The listing builds one solid part. Answer for the finished solid, in the listing's coordinates (mm). A direction names the side the tool comes from. Coordinates: 2 decimals unless noted, no trailing zeros.
from build123d import *

# Parameters (mm, degrees)
F0_W     = 76.2
F0_H     = 76.2
F1_DEPTH = 76.2
F2_W     = 76.2
F2_H     = 76.2
F3_DEPTH = 25.4
F4_W     = 101.6
F4_H     = 76.2
F5_DEPTH = 25.4
F6_W     = 101.6
F6_H     = 101.6
F7_DEPTH = 25.4


with BuildPart() as f1:
    # F0 (on Front) → F1 (new body)
    with BuildSketch(Plane.XZ):
        with Locations((-4.5091081411, 9.3812153666)):
            Rectangle(F0_W, F0_H)
    extrude(amount=F1_DEPTH)

    # F2 (on face) → F3 (join)
    with BuildSketch(Plane.YZ.offset(33.5908918589)):
        with Locations((-38.1, 9.3812153666)):
            Rectangle(F2_W, F2_H)
        with BuildLine():
            Line((-40.5894218998, 3.1841353355), (-54.3512732325, 3.1841353355))
            Line((-54.3512732325, 3.1841353355), (-54.3512732325, -24.2241639644))
            Line((-54.3512732325, -24.2241639644), (-62.0111716158, -24.2241639644))
            Line((-62.0111716158, -24.2241639644), (-62.0111716158, 41.6855831415))
            Line((-62.0111716158, 41.6855831415), (-43.9361194985, 41.6855831415))
            add(Edge.make_bspline(
                [(-43.9361194985, 41.6855831415), (-31.8043407032, 41.6855831415), (-26.0125342985, 37.0405976812)],
                knots=[0, 0, 0, 1, 1, 1], degree=2))
            add(Edge.make_bspline(
                [(-26.0125342985, 37.0405976812), (-20.2207278938, 32.3956122209), (-20.2207278938, 23.0623650382)],
                knots=[0, 0, 0, 1, 1, 1], degree=2))
            add(Edge.make_bspline(
                [(-20.2207278938, 23.0623650382), (-20.2207278938, 9.9929338984), (-33.4776895025, 5.3912247002)],
                knots=[0, 0, 0, 1, 1, 1], degree=2))
            Line((-33.4776895025, 5.3912247002), (-15.5757424335, -24.2241639644))
            Line((-15.5757424335, -24.2241639644), (-24.6349066232, -24.2241639644))
            Line((-24.6349066232, -24.2241639644), (-40.5894218998, 3.1841353355))
        make_face(mode=Mode.SUBTRACT)
    extrude(amount=F3_DEPTH)

    # F4 (on face) → F5 (join)
    with BuildSketch(Plane.XZ.offset(76.2)):
        with Locations((8.1908918589, 9.3812153666)):
            Rectangle(F4_W, F4_H)
        Polygon((19.8698597014, -23.9472966641), (12.0777951104, -23.9472966641), (4.0165501062, -3.3620787536), (-21.9239412868, -3.3620787536), (-29.8860145599, -23.9472966641), (-37.5080704689, -23.9472966641), (-11.92176383, 41.0526894153), (-5.588940426, 41.0526894153), align=None, mode=Mode.SUBTRACT)
    extrude(amount=F5_DEPTH)

    # F6 (on face) → F7 (join)
    with BuildSketch(Plane.XY.offset(47.4812153666)):
        with Locations((8.1908918589, -50.8)):
            Rectangle(F6_W, F6_H)
        with BuildLine():
            add(Edge.make_bspline(
                [(28.9588458513, -20.3443608997), (19.3893672711, -15.8638535876), (9.8198886909, -15.8638535876)],
                knots=[0, 0, 0, 1, 1, 1], degree=2))
            add(Edge.make_bspline(
                [(9.8198886909, -15.8638535876), (-4.0641524861, -15.8638535876), (-12.1032520256, -25.1106618881)],
                knots=[0, 0, 0, 1, 1, 1], degree=2))
            add(Edge.make_bspline(
                [(-12.1032520256, -25.1106618881), (-20.142351565, -34.3574701886), (-20.142351565, -50.4356692674)],
                knots=[0, 0, 0, 1, 1, 1], degree=2))
            add(Edge.make_bspline(
                [(-20.142351565, -50.4356692674), (-20.142351565, -66.956387587), (-12.3890457018, -75.9819362672)],
                knots=[0, 0, 0, 1, 1, 1], degree=2))
            add(Edge.make_bspline(
                [(-12.3890457018, -75.9819362672), (-4.6357398387, -85.0074849473), (9.7092588807, -85.0074849473)],
                knots=[0, 0, 0, 1, 1, 1], degree=2))
            add(Edge.make_bspline(
                [(9.7092588807, -85.0074849473), (18.5227670914, -85.0074849473), (29.825446031, -81.8360970556)],
                knots=[0, 0, 0, 1, 1, 1], degree=2))
            Line((29.825446031, -81.8360970556), (29.825446031, -90.4099073442))
            add(Edge.make_bspline(
                [(29.825446031, -90.4099073442), (21.0672527254, -93.7103633478), (8.2157564434, -93.7103633478)],
                knots=[0, 0, 0, 1, 1, 1], degree=2))
            add(Edge.make_bspline(
                [(8.2157564434, -93.7103633478), (-10.3884899678, -93.7103633478), (-20.501898448, -82.4076844082)],
                knots=[0, 0, 0, 1, 1, 1], degree=2))
            add(Edge.make_bspline(
                [(-20.501898448, -82.4076844082), (-30.6153069283, -71.1050054686), (-30.6153069283, -50.3066011556)],
                knots=[0, 0, 0, 1, 1, 1], degree=2))
            add(Edge.make_bspline(
                [(-30.6153069283, -50.3066011556), (-30.6153069283, -37.2891601583), (-25.7475952805, -27.4984219577)],
                knots=[0, 0, 0, 1, 1, 1], degree=2))
            add(Edge.make_bspline(
                [(-25.7475952805, -27.4984219577), (-20.8798836328, -17.7076837572), (-11.6883902374, -12.4066720196)],
                knots=[0, 0, 0, 1, 1, 1], degree=2))
            add(Edge.make_bspline(
                [(-11.6883902374, -12.4066720196), (-2.496896842, -7.105660282), (9.9489568028, -7.105660282)],
                knots=[0, 0, 0, 1, 1, 1], degree=2))
            add(Edge.make_bspline(
                [(9.9489568028, -7.105660282), (23.1876574204, -7.105660282), (33.1074637329, -11.9364953264)],
                knots=[0, 0, 0, 1, 1, 1], degree=2))
            Line((33.1074637329, -11.9364953264), (28.9588458513, -20.3443608997))
        make_face(mode=Mode.SUBTRACT)
    extrude(amount=F7_DEPTH)


solid = f1.part
Q1. Determine the mould class of faces 6 (the face through (7, -101.6, 21)), 7 (the face through (-20, -44, 47.481)), 8 (the face through (-9, -89, 41.053)), 9 (the face through (46.11, -32.5, -10.71)) for opening direction Z: released by +Z, released by -Z, zero draft, split by the parting line, or undercut.
Answers below:
face 6: zero draft
face 7: released by +Z
face 8: undercut
face 9: undercut
Q2. Which of the six approach directions +Z, -Z, +X, -X, +Y, -Y give full straight-line access (tool end or side, diameter ignored) to faces 1 (the face through (-42.609, -52, 21)), 2 (the face through (46, -20, -24.224)), 3 (the face through (-9, -89, -3.362)), 4 (the face through (31.062, -16.082, 60.003)), 5 (the face through (58.991, -63, 21))?
Answers below:
face 1: +Z, -Z, -X, +Y, -Y
face 2: +X
face 3: -Y
face 4: +Z
face 5: +Z, -Z, +X, +Y, -Y
Q3. Find the intervals of material crossed by probe 1 along Z at (x, y) = (49, -53.5); probe 2 along Z at (x, y) = (-25.5, -65); probe 3 along Y at (x, z) = (35, 3), in increasing order.
Answers below:
probe 1: z = -28.72 to 3.18, 41.69 to 72.88
probe 2: z = -28.72 to 47.48
probe 3: y = -101.6 to -62.01, -54.35 to -40.48, -32.03 to 0
